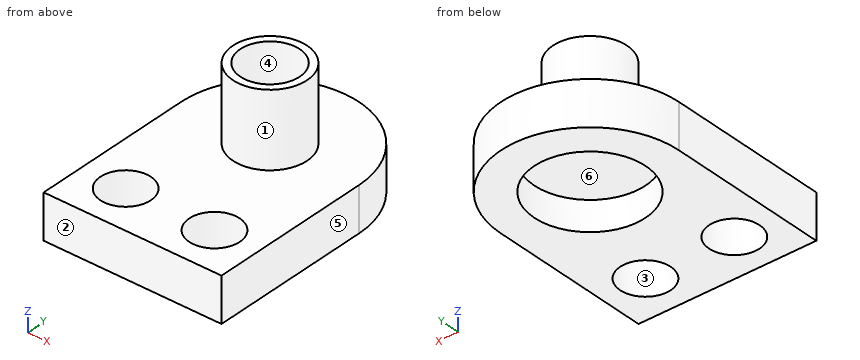
Solid Edge part; units mm, degrees
sketch "Sketch1" plane through (0, 0, 0) normal (0, 0, 1) x (1, 0, 0)
  line L0 (5.9995, 0) -> (5.9995, -11)
  line L1 (-5.9984, -11) -> (5.9995, -11)
  line L2 (-5.9995, -0.0006) -> (-5.9984, -11)
  arc A0 (-5.9995, -0.0006) -> (5.9995, 0) centre (0, 0) cw
  circle A1 centre (-2.9987, -8) radius 1.7
  circle A2 centre (2.9995, -8) radius 1.7
extrude "Protrusion1" add sketch "Sketch1" along normal blind 1
sketch "Sketch2" plane through (0, 0, 0) normal (0, 0, 1) x (1, 0, 0)
  line L0 (5.9995, 0) -> (5.9995, -11)
  line L1 (-5.9984, -11) -> (5.9995, -11)
  line L2 (-5.9995, -0.0006) -> (-5.9984, -11)
  arc A0 (-5.9995, -0.0006) -> (5.9995, 0) centre (0, 0) cw
  circle A1 centre (0, 0) radius 3.75
  circle A2 centre (2.9995, -8) radius 1.7
  circle A3 centre (-2.9987, -8) radius 1.7
extrude "ExtrudedProtrusion_3" add sketch "Sketch2" against normal blind 2
sketch "Sketch3" plane through (0, -2.5002, 1) normal (0, 0, 1) x (1, 0, 0)
  circle A0 centre (0, 2.5002) radius 2.5
  circle A1 centre (0, 2.5002) radius 2
extrude "ExtrudedProtrusion_4" add sketch "Sketch3" along normal blind 5
Verification items for the finished model (mm, model axes). Face numbers are marked on the shaded views. A direction names the side the tool comes from. Round coordinates to 2 decimals unless told otherwise and drop trailing zeros. Order: outer loops, then holes, each group sorted by start corner. A loop starts at its lowest first (then second) coordinate and runs counter-clockwise, first axis right, second up. Notation, with made-up numbers: (84.25, 28.5) - (101.25, 28.5) arc R25 cw to (101.25, 42.5) - close; hole circle Ø8 at (12.5, 27.25). An arc over 180 degrees is marked (long way). Use CSV: the item, a comma, the result in double quotes.
(1) Section check D-D on x = 0. Record the boundary of the cut face in (y, z).
Entries:
outline,"(-11, -2) - (-3.75, -2) - (-3.75, 0) - (3.75, 0) - (3.75, -2) - (6, -2) - (6, 1) - (2.5, 1) - (2.5, 6) - (2, 6) - (2, 1) - (-2, 1) - (-2, 6) - (-2.5, 6) - (-2.5, 1) - (-11, 1) - close"
(2) Section check A-A on z = -1.25. Record the boundary of the cut face in (x, y).
Entries:
outline,"(-6, -11) - (6, -11) - (6, 0) arc R6 ccw to (-6, 0) - close; hole circle Ø3.4 at (-3, -8); hole circle Ø7.5 at (0, 0); hole circle Ø3.4 at (3, -8)"
(3) Gauge pin test, flat ends, axial feed: pin 1 Ø1.5 at (x, y) = (-2.5, 3) entering from +Z; pin 2 Ø3 at (x, z) = (2.5, 0.5) entering from +Y; pin 3 Ø3 at (x, y) = (-3, -8) entering from -Z; pin 4 Ø6.5 at (x, y) = (0, 0) entering from -Z. Record the tip position at first contact, or that the pin passes through.
Entries:
pin 1,"z = 1"
pin 2,"y = 5.92"
pin 3,"through"
pin 4,"z = 0"
(4) Mould release check, pull along Y, two halves, no side actions. Record for the marked faces 1, 2 and 3: released by +Y, released by -Y, zero draft, split by the parting line, or undercut.
Entries:
face 1,"split by the parting line"
face 2,"released by -Y"
face 3,"undercut"
(5) Section check C-C on y = -8. Record the boundary of the cut face in (x, z), and give its area (3 significant figures).
Entries:
outline,"(-6, -2) - (-4.7, -2) - (-4.7, 1) - (-6, 1) - close; (-1.3, -2) - (1.3, -2) - (1.3, 1) - (-1.3, 1) - close; (4.7, -2) - (6, -2) - (6, 1) - (4.7, 1) - close"
area,"15.6 mm^2"
(6) Access from +Z, -Z, +X, -X, +Y, -Y to the whole of each face (thin tool, end or side, straight path). Record for the marked faces 4, 5 and 6.
Entries:
face 4,"+Z"
face 5,"+Z, -Z, +X, +Y, -Y"
face 6,"-Z"
(7) Thickness scan on probe 1 along Z at (x, y) = (5, -5.25); probe 2 along Z at (x, y) = (-1.25, 2); probe 3 along Y at (x, z) = (1.5, 1.75). Record the ranges inside material, lowest first. Write a range as from..to.
Entries:
probe 1,"-2..1"
probe 2,"0..6"
probe 3,"-2..-1.32, 1.32..2"
(8) Section check B-B on x = -4.5. Record the boundary of the cut face in (y, z), and give its area (3 significant figures).
Entries:
outline,"(-11, -2) - (-8.8, -2) - (-8.8, 1) - (-11, 1) - close; (-7.2, -2) - (3.97, -2) - (3.97, 1) - (-7.2, 1) - close"
area,"40.1 mm^2"
